The model under review builds one solid part; all positions refer to its coordinate system, in mm. Round coordinates to 2 decimals unless told otherwise and drop trailing zeros. Order: outer loops, then holes, each group sorted by start corner. A loop starts at its lowest first (then second) coordinate and runs counter-clockwise, first axis right, second up. Notation, with made-up numbers: M -38.75,60.5 L 18.25,60.5 A24 ccw 18.25,73.5 Z; hole C 17.5,-26.75 d9. An arc over 180 degrees is marked long. Answer as a JSON object with one key per item and string values. Group by question number.
1. Add section A-A on z = -2. State the section outline as (x, y) points.
2. Add section D-D on x = -168. State the section outline as (y, z) points.
3. To check wall thickness, follow probe 1 along Y at (x, z) = (0, 0.75); probe 2 along Y at (x, z) = (-564, -3.25); probe 3 along X at (y, z) = (-552.5, 1.75). State the ranges of each line that lie inside material, in increasing order. Write a range as [from, to].
4. Add section C-C on y = -130. State the section outline as (x, z) points, and give its area (3 significant figures).
5. Clearance check with a flat-ended pin moving along its axis: P1, Ø3, axis at y = -333, z = -1.5, coming from the -X side. State where the tip first meets the part, or that it passes through.
6. Add section B-B on x = -50. State the section outline as (y, z) points, and give its area (3 significant figures).
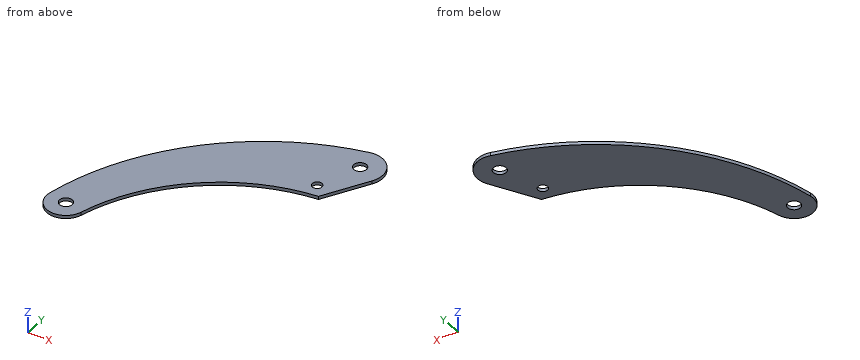
```python
from build123d import *

# Parameters (mm, degrees)
SKETCH1_R           = 20
SKETCH1_R_2         = 15
BOSS_EXTRUDE1_DEPTH = 5


with BuildPart() as part:
    # Sketch1 → Boss-Extrude1 (new body, symmetric)
    with BuildSketch(Plane.XY):
        with BuildLine():
            Line((60.220407354, -35.686167321), (-19.779592646, -170.686167321))
            ThreePointArc((-19.779592646, -170.686167321), (-322.664914871, -293.556077803), (-502.341900983, -566.599506551))
            ThreePointArc((-502.341900983, -566.599506551), (-574.483190404, -608.225743411), (-618.715737076, -537.652440745))
            ThreePointArc((-618.715737076, -537.652440745), (-406.524759245, -145.05016338), (-14.634584071, 68.45311497))
            ThreePointArc((-14.634584071, 68.45311497), (56.839813073, 40.856280421), (60.220407354, -35.686167321))
        make_face()
        Circle(SKETCH1_R, mode=Mode.SUBTRACT)
        with Locations((-50, -130)):
            Circle(SKETCH1_R_2, mode=Mode.SUBTRACT)
        with Locations((-560, -550)):
            Circle(SKETCH1_R, mode=Mode.SUBTRACT)
    extrude(amount=BOSS_EXTRUDE1_DEPTH, both=True)


solid = part.part
```
Recorded:
{
 "1": {"outline": "M -618.72,-537.65 A60 ccw -502.34,-566.6 A550 cw -19.78,-170.69 L 60.22,-35.69 A70 ccw -14.63,68.45 A785 ccw Z; hole C -560,-550 d40; hole C -50,-130 d30; hole C 0,0 d40"},
 "2": {"outline": "M -204.18,-5 L 18.74,-5 L 18.74,5 L -204.18,5 Z"},
 "3": {"probe 1": "y = [-137.31, -20], [20, 70]", "probe 2": "y = [-609.87, -569.6], [-530.4, -371.83]", "probe 3": "x = [-619.95, -579.84], [-540.16, -498.08]"},
 "4": {"outline": "M -391.11,-5 L -65,-5 L -65,5 L -391.11,5 Z; M -35,-5 L 4.33,-5 L 4.33,5 L -35,5 Z", "area": "3,650 mm²"},
 "5": {"P1": "stops at x = -545.66"},
 "6": {"outline": "M -174.06,-5 L -145,-5 L -145,5 L -174.06,5 Z; M -115,-5 L 60.03,-5 L 60.03,5 L -115,5 Z", "area": "2,040 mm²"}
}
